from build123d import *

# Parameters (mm, degrees)
SKETCH1_W           = 200
SKETCH1_H           = 27
BOSS_EXTRUDE1_DEPTH = 1
SKETCH2_W           = 200
SKETCH2_H           = 3.5
BOSS_EXTRUDE2_DEPTH = 6.75
SKETCH3_R           = 2.3
TOP_SLOT_DEPTH      = 102.132648042


with BuildPart() as part:
    # Sketch1 → Boss-Extrude1 (new body)
    with BuildSketch(Plane.XY):
        Rectangle(SKETCH1_W, SKETCH1_H)
    extrude(amount=-BOSS_EXTRUDE1_DEPTH)

    # Sketch2 → Boss-Extrude2 (add)
    with BuildSketch(Plane.XY):
        with Locations((0, 11.75)):
            Rectangle(SKETCH2_W, SKETCH2_H)
        with Locations((0, -11.75)):
            Rectangle(SKETCH2_W, SKETCH2_H)
    extrude(amount=BOSS_EXTRUDE2_DEPTH)

    # Sketch3 → Top Slot (cut, symmetric)
    with BuildSketch(Plane(origin=(0, 0, 0), x_dir=(0, 0, -1), z_dir=(1, 0, 0))):
        with Locations((-4.75, 9.5)):
            Circle(SKETCH3_R)
    top_slot = extrude(amount=TOP_SLOT_DEPTH, both=True, mode=Mode.SUBTRACT)

    # Bottom Slot: Top Slot across plane
    add(top_slot.mirror(Plane.ZX), mode=Mode.SUBTRACT)


solid = part.part
Read the model definition and answer for the solid it produces. Units are mm, in the model's axes. A direction names the side the tool comes from. Coordinates: 2 decimals unless noted, no trailing zeros. Loops run counter-clockwise (first coordinate to the right, second up) from the corner with the lowest first, then second, coordinate; pieces in that order, holes last. Notation, with made-up numbers: (-21, -29) -> (3, -29) arc R16 ccw to (3, 2) -> close; hole circle Ø7 at (5.5, 30.25). An arc over 180 degrees is marked (long way). Answer in a Markdown table with one row per item.
Item 1: For a pull along Y with two mould halves and no side action, classify faces 1 (the flat face through (-1, -13.5, 3)), 2 (the flat face through (-100, -0.1, -0.3)), 3 (the cylindrical face through (1.4, 11.77, 4.37)) as released by +Y, released by -Y, zero draft, split by the parting line, or undercut.
Returned:
| item | result |
|---|---|
| face 1 | released by -Y |
| face 2 | zero draft |
| face 3 | undercut |
Item 2: A cutting plane is placed at B-B on x = -76. Determine the outline of the cut face in (y, z) (3 decimals), plus the area to 3 significant figures.
Returned:
| item | result |
|---|---|
| outline | (-13.5, -1) -> (13.5, -1) -> (13.5, 6.75) -> (10.636, 6.75) arc R2.3 cw to (10, 2.505) -> (10, 0) -> (-10, 0) -> (-10, 2.505) arc R2.3 cw to (-10.636, 6.75) -> (-13.5, 6.75) -> close |
| area | 62.4 mm^2 |
Item 3: This flat-tipped pin is pushed along its axis until it touches: P1, Ø1, axis at x = -7, y = 6.5, coming from the +Z side. Where does it stop, or does it pass through?
Returned:
| item | result |
|---|---|
| P1 | stops at z = 0 |
Item 4: A cutting plane is placed at C-C on y = -5. Determine the outline of the cut face in (x, z), plus the area to 3 significant figures.
Returned:
| item | result |
|---|---|
| outline | (-100, -1) -> (100, -1) -> (100, 0) -> (-100, 0) -> close |
| area | 200 mm^2 |
Item 5: A cutting plane is placed at A-A on z = 4.75. Determine the outline of the cut face in (x, y).
Returned:
| item | result |
|---|---|
| outline | (-100, -13.5) -> (100, -13.5) -> (100, -11.8) -> (-100, -11.8) -> close; (-100, 11.8) -> (100, 11.8) -> (100, 13.5) -> (-100, 13.5) -> close |
Item 6: Straight lines are drawn through the part: line 1 along Y through (x, z) = (-69, 1.5); line 2 along Y through (x, z) = (-62, 5); line 3 along Z through (x, y) = (45, -6). For each, find the intervals that lie inside material, in ascending order. Write a range as [from, to].
Returned:
| item | result |
|---|---|
| line 1 | y = [-13.5, -10], [10, 13.5] |
| line 2 | y = [-13.5, -11.79], [11.79, 13.5] |
| line 3 | z = [-1, 0] |
Item 7: For faces 4 (the cylindrical face through (1.4, -11.77, 4.37)), 5 (the flat face through (-1, 0, 0)), 6 (the flat face through (-1, 0, -1)), determine the directions among +Z, -Z, +X, -X, +Y, -Y from which every point of the face is accessible in a straight line to the end or side of a thin tool.
Returned:
| item | result |
|---|---|
| face 4 | +X, -X |
| face 5 | +Z, +X, -X |
| face 6 | -Z, +X, -X, +Y, -Y |
